Can you work these out from the model? Positions are in its coordinate system, mm. A direction names the side the tool comes from. Coordinates: 2 decimals unless noted, no trailing zeros. Order: outer loops, then holes, each group sorted by start corner. A loop starts at its lowest first (then second) coordinate and runs counter-clockwise, first axis right, second up. Notation, with made-up numbers: (-33, -26) -> (-14, -26) arc R37 cw to (-14, 11) -> close; hole circle Ø9 at (67.5, -37). An arc over 180 degrees is marked (long way). Answer as CSV lines item,"result".
from build123d import *
from build123d.topology import SkipClean

# Parameters (mm, degrees)
SKIZZE1_R                       = 12
SKIZZE1_R_2                     = 1.5
AUFSATZ_LINEAR_AUSTRAGEN1_DEPTH = 18
AUFSATZ_LINEAR_START            = 1
SKIZZE4_R                       = 15
SKIZZE4_R_2                     = 1.5
AUFSATZ_LINEAR_AUSTRAGEN2_DEPTH = 1
SKIZZE2_R                       = 2.9
SCHNITT_LINEAR_AUSTRAGEN4_DEPTH = 14
SCHNITT_LINEAR_AUSTRAGEN5_DEPTH = 23
SKIZZE9_R                       = 2.5
SCHNITT_LINEAR_AUSTRAGEN7_DEPTH = 5
SKIZZE11_R                      = 6
SCHNITT_LINEAR_AUSTRAGEN9_DEPTH = 20


with BuildPart() as part:
    # Skizze1 → Aufsatz-Linear austragen1 (new body)
    with BuildSketch(Plane.XY):
        Circle(SKIZZE1_R)
        with Locations((9, 0)):
            Circle(SKIZZE1_R_2, mode=Mode.SUBTRACT)
        with Locations((0, -9)):
            Circle(SKIZZE1_R_2, mode=Mode.SUBTRACT)
        with Locations((-9, 0)):
            Circle(SKIZZE1_R_2, mode=Mode.SUBTRACT)
        with Locations((0, 9)):
            Circle(SKIZZE1_R_2, mode=Mode.SUBTRACT)
    extrude(amount=AUFSATZ_LINEAR_AUSTRAGEN1_DEPTH)

    # Skizze4 → Aufsatz-Linear austragen2 (add)
    with SkipClean():  # the faces are left unmerged after this step: merging them gives an invalid solid
        with BuildSketch(Plane(origin=(0, 0, 0), x_dir=(-1, 0, 0), z_dir=(0, 0, -1)).offset(AUFSATZ_LINEAR_START)):
            Circle(SKIZZE4_R)
            with Locations((0, 9)):
                Circle(SKIZZE4_R_2, mode=Mode.SUBTRACT)
            with Locations((9, 0)):
                Circle(SKIZZE4_R_2, mode=Mode.SUBTRACT)
            with Locations((0, -9)):
                Circle(SKIZZE4_R_2, mode=Mode.SUBTRACT)
            with Locations((-9, 0)):
                Circle(SKIZZE4_R_2, mode=Mode.SUBTRACT)
        extrude(amount=-AUFSATZ_LINEAR_AUSTRAGEN2_DEPTH)

    # Skizze2 → Schnitt-Linear austragen4 (cut)
    with BuildSketch(Plane.XY.offset(18)):
        with Locations((0, 9)):
            Circle(SKIZZE2_R)
        with Locations((9, 0)):
            Circle(SKIZZE2_R)
        with Locations((0, -9)):
            Circle(SKIZZE2_R)
        with Locations((-9, 0)):
            Circle(SKIZZE2_R)
    extrude(amount=-SCHNITT_LINEAR_AUSTRAGEN4_DEPTH, mode=Mode.SUBTRACT)

    # Skizze6 → Schnitt-Linear austragen5 (cut)
    with BuildSketch(Plane.XY.offset(18)):
        with BuildLine():
            Line((1.5, 2), (-1.5, 2))
            ThreePointArc((-1.5, 2), (-1.118033989, -2.236067977), (2.5, 0))
            ThreePointArc((2.5, 0), (2.236067977, 1.118033989), (1.5, 2))
        make_face()
    extrude(amount=-SCHNITT_LINEAR_AUSTRAGEN5_DEPTH, mode=Mode.SUBTRACT)

    # Skizze9 → Schnitt-Linear austragen7 (cut)
    with BuildSketch(Plane.XY.offset(18)):
        Circle(SKIZZE9_R)
    extrude(amount=-SCHNITT_LINEAR_AUSTRAGEN7_DEPTH, mode=Mode.SUBTRACT)

    # Skizze11 → Schnitt-Linear austragen9 (cut)
    with BuildSketch(Plane.XY.offset(18)):
        Circle(SKIZZE11_R)
    extrude(amount=-SCHNITT_LINEAR_AUSTRAGEN9_DEPTH, mode=Mode.SUBTRACT)


solid = part.part
Q1. Imagine slicing it at C-C (z = 16). List the corners of the cut face in (x, y) for me.
Solution:
outline,"circle Ø24 at (0, 0); hole circle Ø5.8 at (-9, 0); hole circle Ø12 at (0, 0); hole circle Ø5.8 at (0, -9); hole circle Ø5.8 at (0, 9); hole circle Ø5.8 at (9, 0)"
Q2. Which directions (+Z, -Z, +X, -X, +Y, -Y) give clear straight access to the entire face, cutting with the end or side of a thin tool? Please do faces 1 (the cylindrical face through (-4.76, -3.65, 8.63)), 2 (the cylindrical face through (6.699, -1.765, 11.098)).
Solution:
face 1,"+Z, -Z"
face 2,"+Z"
Q3. We'd pull the mould along Y, two halves only. Please class faces 3 (the cylindrical face through (1.559, -6.555, 11.098)), 4 (the cylindrical face through (14.985, 0.66, -0.507)), 5 (the flat face through (7, 10, 0)): pulls with the +Y half, pulls with the -Y half, needs draft (parallel to the pull), parting line crosses it, or undercut.
Solution:
face 3,"undercut"
face 4,"parting line crosses it"
face 5,"needs draft"
Q4. If I drill on line 1 (Y direction, x = 0, z = 1.45); line 2 (Y direction, x = -1, z = 14.75); line 3 (Z direction, x = -1.5, y = 8.25), over which ranges is the centre line in solid material (lowest first)?
Solution:
line 1,"-12 to -10.5, -7.5 to -6, 6 to 7.5, 10.5 to 12"
line 2,"-11.96 to -11.72, -6.28 to -5.92, 5.92 to 6.28, 11.72 to 11.96"
line 3,"-1 to 4"
Q5. Imagine slicing it at B-B (x = -9). List the corners of the cut face in (y, z) for me.
Solution:
outline,"(-12, -1) -> (-1.5, -1) -> (-1.5, 4) -> (-2.9, 4) -> (-2.9, 18) -> (-7.94, 18) -> (-7.94, 0) -> (-12, 0) -> close; (1.5, -1) -> (12, -1) -> (12, 0) -> (7.94, 0) -> (7.94, 18) -> (2.9, 18) -> (2.9, 4) -> (1.5, 4) -> close"
Q6. Imagine slicing it at A-A (y = 0). List the corners of the cut face in (x, z) for me.
Solution:
outline,"(-15, -1) -> (-10.5, -1) -> (-10.5, 4) -> (-11.9, 4) -> (-11.9, 18) -> (-12, 18) -> (-12, 0) -> (-15, 0) -> close; (-7.5, -1) -> (-6, -1) -> (-6, 18) -> (-6.1, 18) -> (-6.1, 4) -> (-7.5, 4) -> close; (6, -1) -> (7.5, -1) -> (7.5, 4) -> (6.1, 4) -> (6.1, 18) -> (6, 18) -> close; (10.5, -1) -> (15, -1) -> (15, 0) -> (12, 0) -> (12, 18) -> (11.9, 18) -> (11.9, 4) -> (10.5, 4) -> close"
Q7. For P1, Ø1.5, axis at x = -9.5, y = -10.5, coming from the +Z side; P2, Ø3.5, axis at x = 0, y = -9, coming from the +Z side; P3, Ø2.5, axis at x = 0, y = 9, coming from the +Z side; P4, Ø10, axis at x = 9, z = 3.5, coming from the -Y side, each with a flat end and sliding along its axis, tell me the tip position at first contact or that it passes through.
Solution:
P1,"z = 0"
P2,"z = 4"
P3,"through"
P4,"y = -13.98"
